Read the model definition and answer for the solid it produces. Units are mm, in the model's axes. Coordinates: 2 decimals unless noted, no trailing zeros. Order: outer loops, then holes, each group sorted by start corner. A loop starts at its lowest first (then second) coordinate and runs counter-clockwise, first axis right, second up. Notation, with made-up numbers: (-33, 19.5) - (-26, 19.5) arc R28 ccw to (-26, 48.5) - close; hole circle Ø5 at (4, -33). An arc over 180 degrees is marked (long way). Use one line per item in the form item = value.
```python
from build123d import *

# Parameters (mm, degrees)
SKETCH1_W           = 20
SKETCH1_H           = 11
BOSS_EXTRUDE1_DEPTH = 1.5
SKETCH2_R           = 1.2
CUT_EXTRUDE1_DEPTH  = 1.5


with BuildPart() as part:
    # Sketch1 → Boss-Extrude1 (new body)
    with BuildSketch(Plane(origin=(0, 0, 0), x_dir=(1, 0, 0), z_dir=(0, 1, 0))):
        with Locations((-10, 0)):
            Rectangle(SKETCH1_W, SKETCH1_H)
    extrude(amount=-BOSS_EXTRUDE1_DEPTH)

    # Sketch2 → Cut-Extrude1 (cut)
    with BuildSketch(Plane(origin=(0, 0, 0), x_dir=(1, 0, 0), z_dir=(0, 1, 0))):
        with Locations(Location((-6, 0, 0), (0, 0, 270))):
            Circle(SKETCH2_R)
        with Locations(Location((-14, 0, 0), (0, 0, 270))):
            Circle(SKETCH2_R)
    extrude(amount=-CUT_EXTRUDE1_DEPTH, mode=Mode.SUBTRACT)


solid = part.part
```
(1) Straight lines are drawn through the part: L1, parallel to X at y = -1, z = 0; L2, parallel to Z at x = -15, y = -0.6. For each, find the intervals that lie inside material, in ascending order.
Answer list:
L1 = -20 to -15.2, -12.8 to -7.2, -4.8 to 0
L2 = -5.5 to -0.66, 0.66 to 5.5
(2) The mould has two halves that part along Z. Classify faces 1 (the cylindrical face through (-15.17, -0.74, -0.26)), 2 (the flat face through (-10, -1, 5.5)), 3 (the flat face through (-10, 0, 0)): +Z half, -Z half, draft (parallel to the pull), parting line (faces both ways), or undercut.
Answer list:
face_1 = undercut
face_2 = +Z half
face_3 = draft
(3) Given pin 1 Ø1 at (x, z) = (-17, 0.5) entering from +Y, flat-ended and moving along its own axis, determine where the tip first touches the part or whether it passes through.
Answer list:
pin_1 = 0
(4) Section C-C, the plane y = -1.15 is taken. Write down the section's boundary in (x, z).
Answer list:
outline = (-20, -5.5) - (0, -5.5) - (0, 5.5) - (-20, 5.5) - close; hole circle Ø2.4 at (-14, 0); hole circle Ø2.4 at (-6, 0)
(5) Section A-A, the plane x = -6 is taken. Write down the section's boundary in (y, z).
Answer list:
outline = (-1.5, -5.5) - (0, -5.5) - (0, -1.2) - (-1.5, -1.2) - close; (-1.5, 1.2) - (0, 1.2) - (0, 5.5) - (-1.5, 5.5) - close
(6) Section B-B, the plane z = 0 is taken. Write down the section's boundary in (x, y).
Answer list:
outline = (-20, -1.5) - (-15.2, -1.5) - (-15.2, 0) - (-20, 0) - close; (-12.8, -1.5) - (-7.2, -1.5) - (-7.2, 0) - (-12.8, 0) - close; (-4.8, -1.5) - (0, -1.5) - (0, 0) - (-4.8, 0) - close
